Design review of the part built by this model. Coordinates are the model's own, in mm. A direction names the side the tool comes from. Round coordinates to 2 decimals unless told otherwise and drop trailing zeros. Loops run counter-clockwise (first coordinate to the right, second up) from the corner with the lowest first, then second, coordinate; pieces in that order, holes last. Notation, with made-up numbers: (7.25, 39) - (39.25, 39) arc R34 cw to (39.25, 69) - close; hole circle Ø5 at (-3, -18). An arc over 180 degrees is marked (long way). Use one line per item in the form item = value. Start each with the question number.
(1) We need section D-D, the plane y = 20. Write out the cut boundary in (x, z), then the cut area to 3 significant figures.
(2) Machinability: for faces 1 (the flat face through (21, 25, 0)), 2 (the flat face through (8, 25, 1)), 3 (the flat face through (-0.51, 7.92, -7.72)), 4 (the flat face through (17, -1, -5)), which of the approach directions +Z, -Z, +X, -X, +Y, -Y give a long, thin tool a straight path to every point of the face, cutting with its end or side? Answer none if there is none.
(3) We need section C-C, the plane z = -2. Write out the cut boundary in (x, y), then the cut area to 3 significant figures.
(4) We need section B-B, the plane y = 38.2. Write out the cut boundary in (x, z).
(5) Wall thickness on probe 1 along Y at (x, z) = (33, -5.25); probe 2 along Y at (x, z) = (3, 0.95); probe 3 along X at (y, z) = (17.5, -4.25): over which ranges is each line inside the solid? List them lowest first. Write a range as [from, to].
(6) The part is to be moulded in two halves that separate along X. For faces 5 (the flat face through (-0.5, 21.5, -5.5)), 6 (the flat face through (34.2, 20, -6)), say which applies: released by +X, released by -X, zero draft, split by the parting line, or undercut.
(7) We need section A-A, the plane x = 31.2. Write out the cut boundary in (y, z).
(8) For pin 1 (3 mm diameter, centred on x = 11, y = 20, fed in from -Z); pin 2 (10 mm diameter, centred on x = 22.5, y = 34, fed in from -Z), all flat-tipped, find the tip position at first contact; note any pin that passes through.
from build123d import *

# Parameters (mm, degrees)
SKETCH_W        = 34.2
SKETCH_H        = 41.2
SKETCH_W_2      = 26.2
SKETCH_H_2      = 15
PAD_DEPTH       = 2
SKETCH001_R     = 1.7
POCKET_DEPTH    = 5
SKETCH002_W     = 7.1
SKETCH002_H     = 7.1
POCKET001_DEPTH = 5
SKETCH005_W     = 36.2
SKETCH005_H     = 43.2
SKETCH005_W_2   = 34.2
SKETCH005_H_2   = 41.2
PAD002_DEPTH    = 15
POCKET002_DEPTH = 5


with BuildPart() as part:
    # Sketch → Pad (new body)
    with BuildSketch(Plane.XY):
        with Locations((17.1, 20.6)):
            Rectangle(SKETCH_W, SKETCH_H)
        with Locations((17.1, 15.5)):
            Rectangle(SKETCH_W_2, SKETCH_H_2, mode=Mode.SUBTRACT)
    extrude(amount=PAD_DEPTH)

    # Sketch001 → Pocket (cut)
    with BuildSketch(Plane.XY.offset(2)):
        with Locations((3, 38.2)):
            Circle(SKETCH001_R)
        with Locations((31.2, 38.2)):
            Circle(SKETCH001_R)
    extrude(amount=-POCKET_DEPTH, mode=Mode.SUBTRACT)

    # Sketch002 → Pocket001 (cut)
    with BuildSketch(Plane.XY.offset(2)):
        with Locations((8, 28.55)):
            Rectangle(SKETCH002_W, SKETCH002_H)
        with Locations((17.1, 28.55)):
            Rectangle(SKETCH002_W, SKETCH002_H)
        with Locations((26.2, 28.55)):
            Rectangle(SKETCH002_W, SKETCH002_H)
    extrude(amount=-POCKET001_DEPTH, mode=Mode.SUBTRACT)

    # Sketch005 → Pad002 (new body)
    with BuildSketch(Plane.XY.offset(2)):
        with Locations((17.1, 20.6)):
            Rectangle(SKETCH005_W, SKETCH005_H)
        with Locations((17.1, 20.6)):
            Rectangle(SKETCH005_W_2, SKETCH005_H_2, mode=Mode.SUBTRACT)
    extrude(amount=-PAD002_DEPTH)

    # Sketch006 → Pocket002 (cut)
    with BuildSketch(Plane(origin=(-1, 0, 0), x_dir=(0, -1, 0), z_dir=(-1, 0, 0))):
        Polygon((-5.2, -13), (-32.2, -13), (-32.2, -5.500487), (-10.562311, -5.500487), (-5.2, -10), align=None)
    extrude(amount=-POCKET002_DEPTH, mode=Mode.SUBTRACT)


solid = part.part
Data:
q1.outline = (-1, -5.5) - (0, -5.5) - (0, 0) - (4, 0) - (4, 2) - (-1, 2) - close; (30.2, 0) - (34.2, 0) - (34.2, -13) - (35.2, -13) - (35.2, 2) - (30.2, 2) - close
q1.area = 38.5 mm^2
q2.face_1 = -Z
q2.face_2 = +Z, -Z
q2.face_3 = -Z, -X
q2.face_4 = +Z, -Z, +X, -X, -Y
q3.outline = (-1, -1) - (35.2, -1) - (35.2, 42.2) - (-1, 42.2) - close; hole (0, 0) - (34.2, 0) - (34.2, 41.2) - (0, 41.2) - close
q3.area = 155 mm^2
q4.outline = (-1, -13) - (0, -13) - (0, 0) - (1.3, 0) - (1.3, 2) - (-1, 2) - close; (4.7, 0) - (29.5, 0) - (29.5, 2) - (4.7, 2) - close; (32.9, 0) - (34.2, 0) - (34.2, -13) - (35.2, -13) - (35.2, 2) - (32.9, 2) - close
q5.probe_1 = [-1, 0], [41.2, 42.2]
q5.probe_2 = [-1, 36.5], [39.9, 42.2]
q5.probe_3 = [-1, 0], [34.2, 35.2]
q6.face_5 = zero draft
q6.face_6 = undercut
q7.outline = (-1, -13) - (0, -13) - (0, 0) - (36.5, 0) - (36.5, 2) - (-1, 2) - close; (39.9, 0) - (41.2, 0) - (41.2, -13) - (42.2, -13) - (42.2, 2) - (39.9, 2) - close
q8.pin_1 = through
q8.pin_2 = 0
